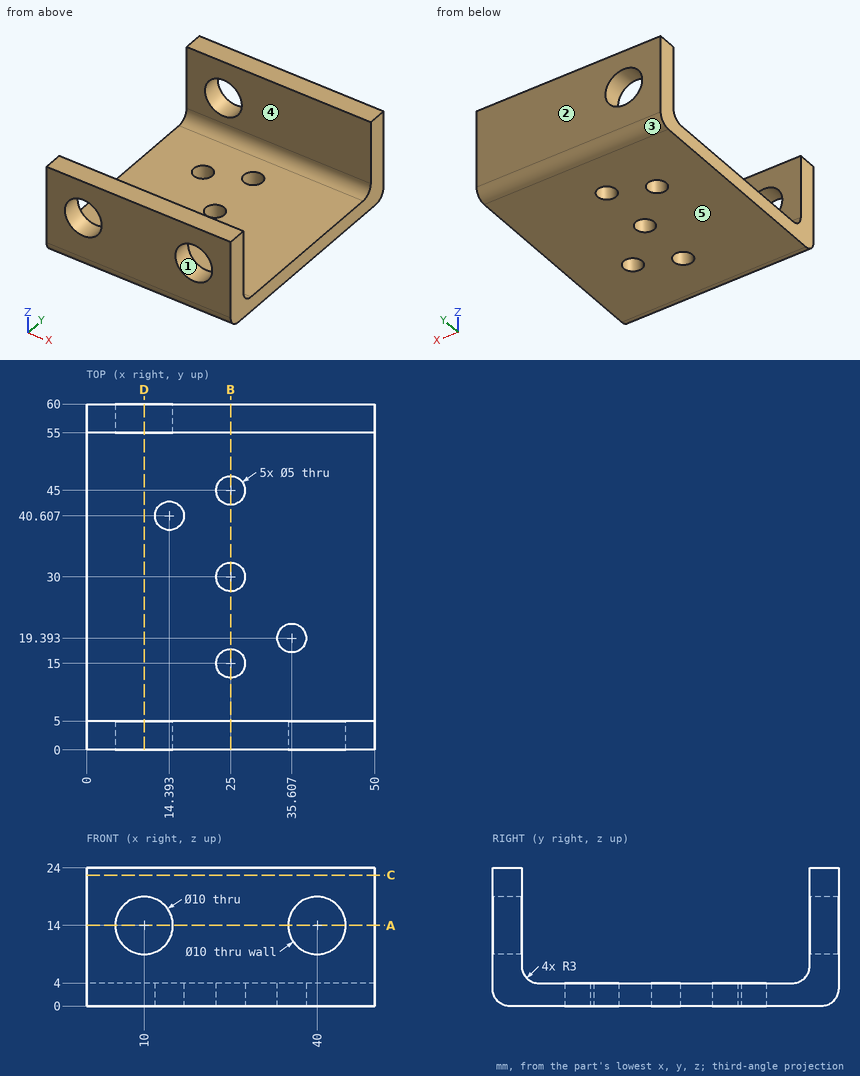
Answer from the drawing. Dimensions are ordinates in mm from the lowest x, y and z of the part. A direction names the side the tool comes from. Coordinates: 2 decimals unless noted, no trailing zeros. Order: outer loops, then holes, each group sorted by start corner. A loop starts at its lowest first (then second) coordinate and runs counter-clockwise, first axis right, second up. Notation, with made-up numbers: (64, 10.5) - (84, 10.5) arc R22 ccw to (84, 26.5) - close; hole circle Ø5 at (32.5, -35). An arc over 180 degrees is marked (long way). Answer as a JSON object with one key per item and string values. Group by question number.
Item 1: Flat-ended cylindrical pins translate along their axes: P1, Ø12, axis at x = 37.5, y = 50.5, coming from the +Z side; P2, Ø22, axis at x = 20, y = 27.5, coming from the +Z side. Find the tip coordinate at first contact, or state that the pin passes through.
Item 2: Section B-B (x = 25) is taken. Give the vertices of the cut face in (y, z).
Item 3: Consider probe 1 along Y at (x, z) = (9, 7.25); probe 2 along Y at (x, z) = (25, 2.15); probe 3 along Z at (x, y) = (10, 57). Determine where each line is inside the solid, lowest interval first. Write a range as from..to.
Item 4: Section D-D (x = 10) is taken. Give the vertices of the cut face in (y, z).
Item 5: Section A-A (z = 14) is taken. Give the vertices of the cut face in (x, y).
Item 6: A tool of negligible diameter and unlimited length cuts with its end or side. For the marked faces 4 and 5, from which of +Z, -Z, +X, -X, +Y, -Y can it reach the whole face along a straight path? Write none if from no direction.
Item 7: Section C-C (z = 22.75) is taken. Give the vertices of the cut face in (x, y).
Item 8: The mould has two halves that part along Z. Classify the marked faces 1, 2 and 3: +Z half, -Z half, draft (parallel to the pull), parting line (faces both ways), or undercut.
Results are:
{
 "1": {"P1": "stops at z = 24", "P2": "stops at z = 4"},
 "2": {"outline": "(0, 3) arc R3 ccw to (3, 0) - (12.5, 0) - (12.5, 4) - (8, 4) arc R3 cw to (5, 7) - (5, 24) - (0, 24) - close; (17.5, 0) - (27.5, 0) - (27.5, 4) - (17.5, 4) - close; (32.5, 0) - (42.5, 0) - (42.5, 4) - (32.5, 4) - close; (47.5, 0) - (57, 0) arc R3 ccw to (60, 3) - (60, 24) - (55, 24) - (55, 7) arc R3 cw to (52, 4) - (47.5, 4) - close"},
 "3": {"probe 1": "y = 0..5, 55..60", "probe 2": "y = 0.12..12.5, 17.5..27.5, 32.5..42.5, 47.5..59.88", "probe 3": "z = 0..9, 19..24"},
 "4": {"outline": "(0, 3) arc R3 ccw to (3, 0) - (57, 0) arc R3 ccw to (60, 3) - (60, 9) - (55, 9) - (55, 7) arc R3 cw to (52, 4) - (8, 4) arc R3 cw to (5, 7) - (5, 9) - (0, 9) - close; (0, 19) - (5, 19) - (5, 24) - (0, 24) - close; (55, 19) - (60, 19) - (60, 24) - (55, 24) - close"},
 "5": {"outline": "(0, 0) - (5, 0) - (5, 5) - (0, 5) - close; (0, 55) - (5, 55) - (5, 60) - (0, 60) - close; (15, 0) - (35, 0) - (35, 5) - (15, 5) - close; (15, 55) - (50, 55) - (50, 60) - (15, 60) - close; (45, 0) - (50, 0) - (50, 5) - (45, 5) - close"},
 "6": {"face 4": "+Z, +X, -X", "face 5": "-Z, +X, -X, +Y, -Y"},
 "7": {"outline": "(0, 0) - (50, 0) - (50, 5) - (0, 5) - close; (0, 55) - (50, 55) - (50, 60) - (0, 60) - close"},
 "8": {"face 1": "undercut", "face 2": "draft", "face 3": "-Z half"}
}
